```python
from build123d import *

# Parameters (mm, degrees)
SKETCH1_W           = 74.22368895
SKETCH1_H           = 68
SKETCH1_W_2         = 37.111844475
SKETCH1_H_2         = 52
SKETCH1_H_3         = 58
BOSS_EXTRUDE1_DEPTH = 70
SKETCH2_R           = 27.5
CUT_EXTRUDE1_DEPTH  = 70
FILLET1_R           = 19
SKETCH3_W           = 33.111844475
SKETCH3_H           = 64.288874977
CUT_EXTRUDE2_DEPTH  = 58
SKETCH5_W           = 50
SKETCH5_H           = 40
CUT_EXTRUDE3_DEPTH  = 58
SKETCH7_W           = 29.516350972
SKETCH7_H           = 18.630296647
CUT_EXTRUDE5_DEPTH  = 58
SKETCH8_W           = 33.111844475
SKETCH8_H           = 2
CUT_EXTRUDE6_DEPTH  = 58
SKETCH9_W           = 1.55
SKETCH9_H           = 66.288874977
BOSS_EXTRUDE2_DEPTH = 58
SKETCH10_W          = 30.011844475
SKETCH10_H          = 0.145
BOSS_EXTRUDE3_DEPTH = 58
SKETCH11_W          = 37.111844475
SKETCH11_H          = 24.941562027
BOSS_EXTRUDE5_DEPTH = 15
FILLET3_R           = 5
FILLET4_R           = 5
FILLET5_R           = 5


with BuildPart() as part:
    # Sketch1 → Boss-Extrude1 (new body)
    with BuildSketch(Plane(origin=(0, 0, 0), x_dir=(1, 0, 0), z_dir=(0, 1, 0))):
        with Locations((-37.111844475, -34)):
            Rectangle(SKETCH1_W, SKETCH1_H)
        with Locations((-37.111844475, -94)):
            Rectangle(SKETCH1_W_2, SKETCH1_H_2)
        with Locations((-37.111844475, -149)):
            Rectangle(SKETCH1_W_2, SKETCH1_H_3)
    extrude(amount=-BOSS_EXTRUDE1_DEPTH)

    # Sketch2 → Cut-Extrude1 (cut)
    with BuildSketch(Plane(origin=(0, 0, 0), x_dir=(1, 0, 0), z_dir=(0, 1, 0))):
        with Locations(Location((-37.111844475, -34, 0), (0, 0, 270))):
            Circle(SKETCH2_R)
    extrude(amount=-CUT_EXTRUDE1_DEPTH, mode=Mode.SUBTRACT)

    # Fillet1
    # the kernel refuses this fillet: 19 mm, written as the material it takes off along each edge
    with BuildSketch(Plane(origin=(0, 47.487024211, 68), x_dir=(0, 0, -1), z_dir=(0, -1, 0))) as fillet1_piece_1:
        with BuildLine():
            CenterArc((18.994809684, -19), FILLET1_R, 90, 88.660731648)
            Line((0, -18.555922237), (-0.379896194, -18.547040682))
            ThreePointArc((-0.379896194, -18.547040682), (-0.38, -9.277961119), (-0.38, 0))
            Line((-0.38, 0), (0, 0.38))
            Line((0, 0.38), (18.994809684, 0.38))
            Line((18.994809684, 0.38), (18.994809684, 0))
        make_face()
    extrude(amount=164.974048421, mode=Mode.SUBTRACT)
    with BuildSketch(Plane(origin=(0, 47.5, 0), x_dir=(-1, 0, 0), z_dir=(0, -1, 0))) as fillet1_piece_2:
        with BuildLine():
            CenterArc((FILLET1_R, -FILLET1_R), FILLET1_R, 90, 90)
            Line((0, -FILLET1_R), (-FILLET1_R * 0.02, -FILLET1_R))
            Line((-FILLET1_R * 0.02, -FILLET1_R), (-FILLET1_R * 0.02, FILLET1_R * 0.02))
            Line((-FILLET1_R * 0.02, FILLET1_R * 0.02), (FILLET1_R, FILLET1_R * 0.02))
            Line((FILLET1_R, FILLET1_R * 0.02), (FILLET1_R, 0))
        make_face()
    extrude(amount=165, mode=Mode.SUBTRACT)
    with BuildSketch(Plane(origin=(-74.22368895, 47.487024211, 68), x_dir=(0, 0, -1), z_dir=(0, -1, 0))) as fillet1_piece_3:
        with BuildLine():
            CenterArc((18.994809684, 19), FILLET1_R, 181.339268352, 88.660731648)
            Line((0, 18.555922237), (-0.379896194, 18.547040682))
            ThreePointArc((-0.379896194, 18.547040682), (-0.38, 9.277961119), (-0.38, 0))
            Line((-0.38, 0), (0, -0.38))
            Line((0, -0.38), (18.994809684, -0.38))
            Line((18.994809684, -0.38), (18.994809684, 0))
        make_face()
    extrude(amount=164.974048421, mode=Mode.SUBTRACT)
    with BuildSketch(Plane(origin=(-74.22368895, 47.5, 0), x_dir=(1, 0, 0), z_dir=(0, -1, 0))) as fillet1_piece_4:
        with BuildLine():
            CenterArc((FILLET1_R, FILLET1_R), FILLET1_R, 180, 90)
            Line((0, FILLET1_R), (-FILLET1_R * 0.02, FILLET1_R))
            Line((-FILLET1_R * 0.02, FILLET1_R), (-FILLET1_R * 0.02, -FILLET1_R * 0.02))
            Line((-FILLET1_R * 0.02, -FILLET1_R * 0.02), (FILLET1_R, -FILLET1_R * 0.02))
            Line((FILLET1_R, -FILLET1_R * 0.02), (FILLET1_R, 0))
        make_face()
    extrude(amount=165, mode=Mode.SUBTRACT)

    # Sketch3 → Cut-Extrude2 (cut)
    with BuildSketch(Plane.XY.offset(178)):
        with Locations((-37.111844475, -35.855562511)):
            Rectangle(SKETCH3_W, SKETCH3_H)
    extrude(amount=-CUT_EXTRUDE2_DEPTH, mode=Mode.SUBTRACT)

    # Sketch5 → Cut-Extrude3 (cut)
    with BuildSketch(Plane.ZY.offset(55.667766712)):
        with Locations((93, -50)):
            Rectangle(SKETCH5_W, SKETCH5_H)
    extrude(amount=-CUT_EXTRUDE3_DEPTH, mode=Mode.SUBTRACT)

    # Sketch7 → Cut-Extrude5 (cut)
    with BuildSketch(Plane(origin=(0, 0, 118), x_dir=(-1, 0, 0), z_dir=(0, 0, -1))):
        with Locations((37.314097723, -50.684851677)):
            Rectangle(SKETCH7_W, SKETCH7_H)
    extrude(amount=-CUT_EXTRUDE5_DEPTH, mode=Mode.SUBTRACT)

    # Sketch8 → Cut-Extrude6 (cut)
    with BuildSketch(Plane.XY.offset(178)):
        with Locations((-37.111844475, -2.711125023)):
            Rectangle(SKETCH8_W, SKETCH8_H)
    extrude(amount=-CUT_EXTRUDE6_DEPTH, mode=Mode.SUBTRACT)

    # Sketch9 → Boss-Extrude2 (add)
    with BuildSketch(Plane.XY.offset(178)):
        with Locations((-52.892766712, -34.855562511)):
            Rectangle(SKETCH9_W, SKETCH9_H)
        with Locations((-21.330922237, -34.855562511)):
            Rectangle(SKETCH9_W, SKETCH9_H)
    extrude(amount=-BOSS_EXTRUDE2_DEPTH)

    # Sketch10 → Boss-Extrude3 (add)
    with BuildSketch(Plane.XY.offset(178)):
        with Locations((-37.111844475, -67.9275)):
            Rectangle(SKETCH10_W, SKETCH10_H)
        with Locations((-37.111844475, -1.783625023)):
            Rectangle(SKETCH10_W, SKETCH10_H)
    extrude(amount=-BOSS_EXTRUDE3_DEPTH)

    # Sketch11 → Boss-Extrude5 (add)
    with BuildSketch(Plane.XY.offset(178)):
        Polygon((-74.611844475, -49.941562027), (-74.611844475, -109.941562027), (0.388155525, -109.941562027), (0.388155525, -49.941562027), (-18.555922237, -49.941562027), (-18.555922237, -54.941562027), (-4.611844475, -54.941562027), (-4.611844475, -104.941562027), (-69.611844475, -104.941562027), (-69.611844475, -54.941562027), (-55.667766712, -54.941562027), (-55.667766712, -49.941562027), align=None)
        with Locations((-37.111844475, -82.470781014)):
            Rectangle(SKETCH11_W, SKETCH11_H)
    extrude(amount=-BOSS_EXTRUDE5_DEPTH)

    # Fillet3
    fillet3_edges = [part.edges().sort_by_distance(p)[0] for p in [
        (-4.611844475, -104.941562027, 170.5),
        (-4.611844475, -54.941562027, 170.5),
        (0.388155525, -49.941562027, 170.5),
        (0.388155525, -109.941562027, 170.5),
        (-74.611844475, -109.941562027, 170.5),
        (-74.611844475, -49.941562027, 170.5),
        (-69.611844475, -54.941562027, 170.5),
        (-69.611844475, -104.941562027, 170.5),
        (-18.555922237, -94.941562027, 170.5),
        (-55.667766712, -94.941562027, 170.5),
    ]]
    fillet(fillet3_edges, radius=FILLET3_R)

    # Fillet4
    fillet4_edges = [part.edges().sort_by_distance(p)[0] for p in [
        (-18.555922237, -54.941562027, 170.5),
        (-55.667766712, -54.941562027, 170.5),
    ]]
    fillet(fillet4_edges, radius=FILLET4_R)

    # Fillet5
    fillet5_edges = [part.edges().sort_by_distance(p)[0] for p in [
        (-18.555922237, -49.941562027, 170.5),
        (-55.667766712, -49.941562027, 170.5),
    ]]
    fillet(fillet5_edges, radius=FILLET5_R)


solid = part.part
```
Work out the finished part from the listing and answer in its coordinate system (mm). A direction names the side the tool comes from. Round coordinates to 2 decimals unless told otherwise and drop trailing zeros. Write each loop counter-clockwise with the first axis right and the second up, starting at its lowest first coordinate (ties: lowest second). Pieces come first, ordered by that corner, then holes. Notation, with made-up numbers: (87.5, 18.5) - (136.5, 18.5) arc R15 ccw to (136.5, 25.5) - close; hole circle Ø11 at (-25, -23). An arc over 180 degrees is marked (long way). Return JSON: item names as keys, results as strings. Group by question number.
Q1. Each of these flat-tipped pins is pushed along its axis until it touches: pin 1 Ø3 at (x, y) = (-39, -22.5) entering from -Z; pin 2 Ø1 at (y, z) = (-54, 119) entering from -X; pin 3 Ø19.5 at (x, y) = (-52, -81) entering from -Z; pin 4 Ø2 at (x, y) = (-65.5, -54.5) entering from -Z. Where does it stop, or does it pass through?
Q2. The mould has two halves that part along Z. Classify faces 1 (the flat face through (-37, -30, 93)), 2 (the flat face through (0, -35, 34)): released by +Z, released by -Z, zero draft, split by the parting line, or undercut.
Q3. Find the intervals of material crossed by L1, parallel to X at y = -95, z = 164.5; L2, parallel to X at y = -34, z = 34; L3, parallel to Y at x = -45, z = 162.5 (3 decimals), in increasing order.
Q4. The part is cut by section C-C on x = -26.5. Write down the section's boundary in (y, z) (3 decimals), then the cut area to 3 significant figures.
Q5. The part is cut by section D-D on y = -77.5. Write down the section's boundary in (x, z), then the cut area to 3 significant figures.
Q6. The part is cut by section B-B on y = -62. Write down the section's boundary in (x, z).
Q7. For faces 3 (the flat face through (-54, -70, 11)), 4 (the flat face through (-12, -54.942, 171)), 5 (the cylindrical face through (-57.094, -48.438, 170.395)), 6 (the flat face through (-37, -104.942, 171)), 7 (the cylindrical face through (-17.13, -48.44, 170.4)), determine the directions among +Z, -Z, +X, -X, +Y, -Y from which every point of the face is accessible in a straight line to the end or side of a thin tool.
Q8. The part is cut by section A-A on z = 34. Write down the section's boundary in (x, y), then the cut area to 3 significant figures.
Solved:
{
 "1": {"pin 1": "z = 0", "pin 2": "x = -55.67", "pin 3": "z = 163", "pin 4": "z = 2.42"},
 "2": {"face 1": "undercut", "face 2": "zero draft"},
 "3": {"L1": "-74.61 to -69.61, -4.61 to 0.39", "L2": "-74.22 to -64.61, -9.61 to 0", "L3": "-70 to -67.855, -1.856 to 0"},
 "4": {"outline": "(-109.942, 163) - (-104.942, 163) - (-104.942, 178) - (-109.942, 178) - close; (-94.942, 163) - (-70, 163) - (-70, 118) - (-60, 118) - (-60, 120) - (-67.855, 120) - (-67.855, 178) - (-94.942, 178) - close; (-70, 0) - (0, 0) - (0, 8.63) - (-70, 8.63) - close; (-70, 59.37) - (0, 59.37) - (0, 178) - (-1.856, 178) - (-1.856, 120) - (-41.37, 120) - (-41.37, 118) - (-30, 118) - (-30, 68) - (-70, 68) - close", "area": "3,490 mm²"},
 "5": {"outline": "(-74.61, 163) - (-69.61, 163) - (-69.61, 178) - (-74.61, 178) - close; (-55.67, 163) - (-18.56, 163) - (-18.56, 178) - (-55.67, 178) - close; (-4.61, 163) - (0.39, 163) - (0.39, 178) - (-4.61, 178) - close", "area": "707 mm²"},
 "6": {"outline": "(-74.61, 163) - (-69.61, 163) - (-69.61, 178) - (-74.61, 178) - close; (-74.22, 19) arc R19 ccw to (-55.22, 0) - (-19, 0) arc R19 ccw to (0, 19) - (0, 49.01) arc R19 ccw to (-18.56, 68) - (-55.67, 68) arc R19 ccw to (-74.22, 49.01) - close; (-55.67, 118) - (-18.56, 118) - (-18.56, 178) - (-22.11, 178) - (-22.11, 120) - (-52.12, 120) - (-52.12, 178) - (-55.67, 178) - close; (-4.61, 163) - (0.39, 163) - (0.39, 178) - (-4.61, 178) - close; hole circle Ø55 at (-37.11, 34)"},
 "7": {"face 3": "-Z, +X, -X, -Y", "face 4": "+Z", "face 5": "+Z, -X, +Y", "face 6": "+Z, -Z", "face 7": "+Z, +X, +Y"},
 "8": {"outline": "(-74.22, -70) - (-64.61, -70) - (-64.61, 0) - (-74.22, 0) - close; (-9.61, -70) - (0, -70) - (0, 0) - (-9.61, 0) - close", "area": "1,350 mm²"}
}
